from build123d import *

# Parameters (mm, degrees)
F1_DEPTH = 25.4
F3_DEPTH = 25.4


# Not quite as in the source:
# - a feature names something its author has since deleted; it is built from what else it names


with BuildPart() as f1:
    # F0 (on Front) → F1 (new body)
    with BuildSketch(Plane.XZ):
        Polygon((11.7880795151, 53.5375215113), (0, 86.6096317768), (-11.7820905356, 53.5432), (-11.7820905356, 0), (-24.8799551113, 14.2439296469), (-24.8799551113, -14.5713714883), (-12.7764736156, -27.6303915451), (-12.7764736156, -39.4159915451), (11.7880795151, -39.4159915451), (11.7880795151, -26.6211631082), (24.8922296689, -14.5713714883), (24.8922296689, 14.2439296469), (11.7880795151, 0), align=None)
    extrude(amount=F1_DEPTH)

    # F2 (on face) → F3 (join)
    with BuildSketch(Plane.XZ.offset(25.4)):
        Polygon((-0.4971447281, -47.3129446821), (-12.7764736156, -55.2061082793), (-0.4912507866, -63.1106432249), (11.7880795151, -55.2136891784), align=None)
        Polygon((11.7880795151, -39.4159915451), (-12.7764736156, -39.4159915451), (-0.4971447281, -47.3129446821), align=None)
        Polygon((-0.4912507866, -63.1106432249), (-12.7764736156, -71.0113868117), (11.7880795151, -71.0113868117), align=None)
        Polygon((11.7880795151, -39.4159915451), (-0.4971447281, -47.3129446821), (11.7880795151, -55.2136891784), align=None)
        Polygon((-0.4971447281, -47.3129446821), (-12.7764736156, -39.4159915451), (-12.7764736156, -55.2061082793), align=None)
        Polygon((11.7880795151, -55.2136891784), (-0.4912507866, -63.1106432249), (11.7880795151, -71.0113868117), align=None)
        Polygon((-0.4912507866, -63.1106432249), (-12.7764736156, -55.2061082793), (-12.7764736156, -71.0113868117), align=None)
    extrude(amount=-F3_DEPTH)


solid = f1.part
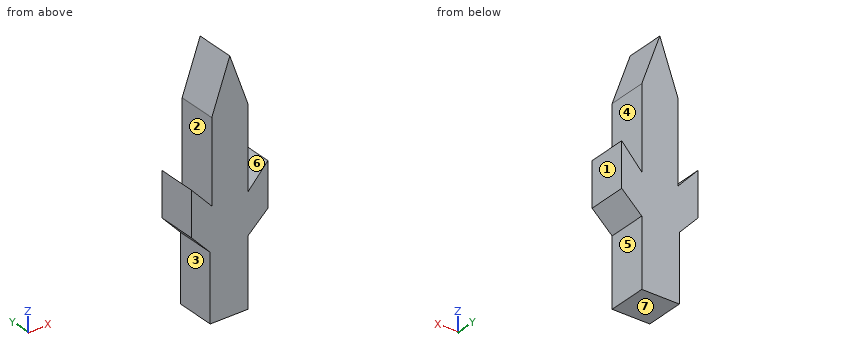
Geometry: final body of the model. Coordinates: model frame, mm. Face numbers are marked on the shaded views. A direction names the side the tool comes from. Coordinates: 2 decimals unless noted, no trailing zeros. Order: outer loops, then holes, each group sorted by start corner. A loop starts at its lowest first (then second) coordinate and runs counter-clockwise, first axis right, second up.
1) Section C-C (x = -4). Return loops of the section in (y, z).
Result sheet:
outline: (-25.4, -71.01) - (0, -71.01) - (0, 75.38) - (-25.4, 75.38) - close
2) First-contact query: P1, Ø7.5, axis at y = -11.5, z = -46, coming from the +X side; P2, Ø12, axis at y = -7, z = -25, coming from the -X side; P3, Ø5, axis at y = -9.5, z = -41.5, coming from the -X side. Flat tips, straight axial feed; report the tip coordinate or a pass-through.
Result sheet:
P1: stops at x = 11.79
P2: stops at x = -20.78
P3: stops at x = -12.78
3) Set-up query: the marked faces 1, 2 and 3. Return all of +Z, -Z, +X, -X, +Y, -Y with unobstructed straight access to the full face (end or side cutting, diameter ignored); none if empty.
Result sheet:
face 1: +Z, -Z, +X, +Y, -Y
face 2: +Z, +Y, -Y
face 3: -Z, -X, +Y, -Y
4) Section A-A (y = -12.25). Return loops of the section in (x, z).
Result sheet:
outline: (-24.88, -14.57) - (-12.78, -27.63) - (-12.78, -71.01) - (11.79, -71.01) - (11.79, -26.62) - (24.89, -14.57) - (24.89, 14.24) - (11.79, 0) - (11.79, 53.54) - (0, 86.61) - (-11.78, 53.54) - (-11.78, 0) - (-24.88, 14.24) - close
5) Section B-B (z = 20.5). Return loops of the section in (x, y), then the cut area to 3 significant figures.
Result sheet:
outline: (-11.78, -25.4) - (11.79, -25.4) - (11.79, 0) - (-11.78, 0) - close
area: 599 mm2
6) Draft query along X for the marked faces 4, 5, 6 and 7. Return one class per face: released by +X, released by -X, zero draft, split by the parting line, or undercut.
Result sheet:
face 4: undercut
face 5: released by +X
face 6: undercut
face 7: zero draft
7) Ray query, probe 1 along X at (y, z) = (-8, 17); probe 2 along X at (y, z) = (-20, -37); probe 3 along Z at (x, y) = (22.5, -16.75). Return the intervals inside material, ascending.
Result sheet:
probe 1: x = -11.78 to 11.79
probe 2: x = -12.78 to 11.79
probe 3: z = -16.77 to 11.64
